Check sheet for the drawn part. Datum: minimum x, y, z corner. Units: mm. A direction names the side the tool comes from. Round coordinates to 2 decimals unless told otherwise and drop trailing zeros. Write each loop counter-clockwise with the first axis right and the second up, starting at its lowest first coordinate (ties: lowest second). Pieces come first, ordered by that corner, then holes. Notation, with made-up numbers: (49.25, -5.5) - (88.25, -5.5) arc R20 cw to (88.25, 31.5) - close; hole circle Ø1 at (27.25, 42.25). An arc over 180 degrees is marked (long way). Write each question's results on one line, items separated by ' | '.
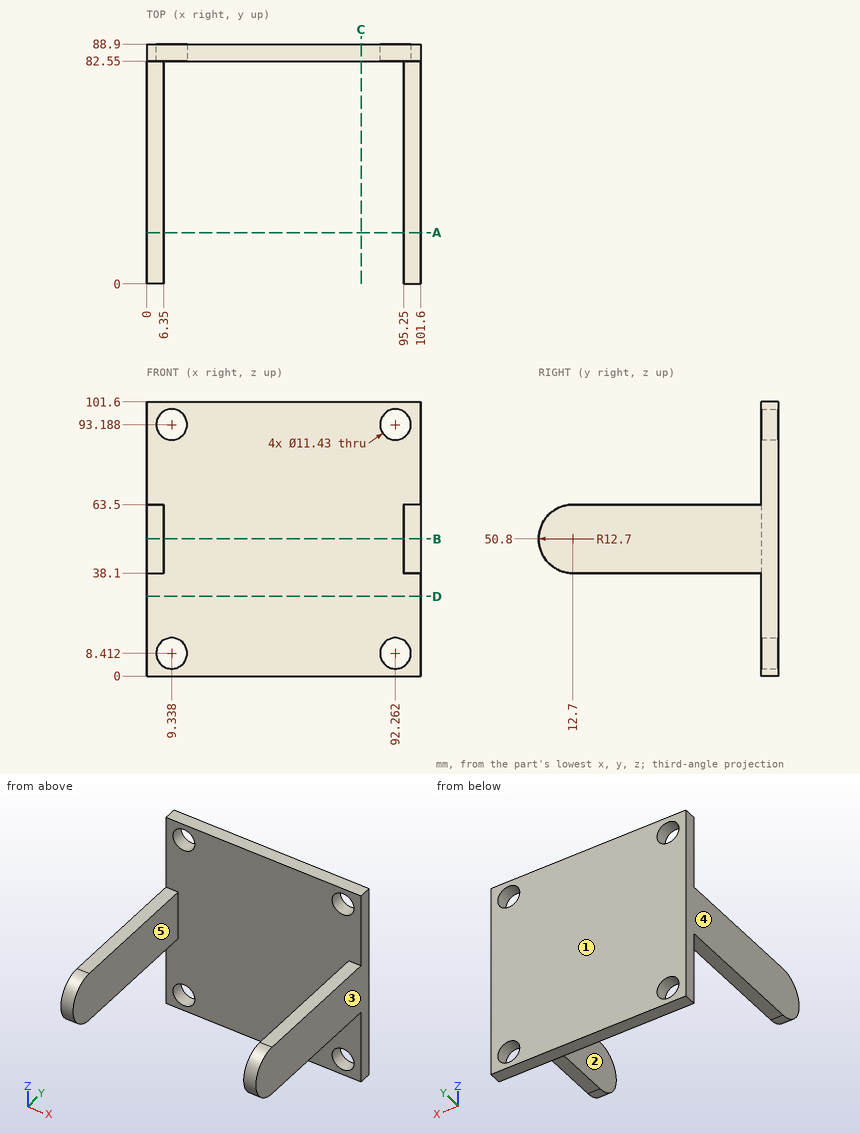
(1) Section check D-D (z = 29.5). Record the cut outline in (x, y), plus the area to 3 significant figures.
Answer:
outline: (0, 82.55) - (101.6, 82.55) - (101.6, 88.9) - (0, 88.9) - close | area: 645 mm2
(2) Thickness scan on L1, parallel to Y at x = 74, z = 12; L2, parallel to X at y = 51, z = 46. Record the ranges inside material, lowest first.
Answer:
L1: 82.55 to 88.9 | L2: 0 to 6.35, 95.25 to 101.6
(3) Set-up check for the marked faces 1 and 2: record each of +Z, -Z, +X, -X, +Y, -Y from which the full face is reachable in a straight line by a thin tool's end or side.
Answer:
face 1: +Z, -Z, +X, -X, +Y | face 2: +Z, -Z, -Y
(4) Mould release check, pull along X, two halves, no side actions. Record for the marked faces 3, 4 and 5: released by +X, released by -X, zero draft, split by the parting line, or undercut.
Answer:
face 3: released by +X | face 4: released by -X | face 5: undercut
(5) Go/stop test with flat-tipped pins: pin 1 Ø2 at (x, z) = (78, 12) entering from -Y; pin 2 Ø7 at (x, y) = (3, 50) entering from -Z; pin 3 Ø3 at (x, y) = (100, 63) entering from +Z. Record where each tip stops, or that it passes through.
Answer:
pin 1: y = 82.55 | pin 2: z = 38.1 | pin 3: z = 63.5
(6) Section check B-B (z = 50.8). Record the cut outline in (x, y).
Answer:
outline: (0, 0) - (6.35, 0) - (6.35, 82.55) - (95.25, 82.55) - (95.25, 0) - (101.6, 0) - (101.6, 88.9) - (0, 88.9) - close
(7) Section check A-A (y = 19). Record the cut outline in (x, z).
Answer:
outline: (0, 38.1) - (6.35, 38.1) - (6.35, 63.5) - (0, 63.5) - close; (95.25, 38.1) - (101.6, 38.1) - (101.6, 63.5) - (95.25, 63.5) - close
(8) Section check C-C (x = 79.5). Record the cut outline in (y, z).
Answer:
outline: (82.55, 0) - (88.9, 0) - (88.9, 101.6) - (82.55, 101.6) - close
